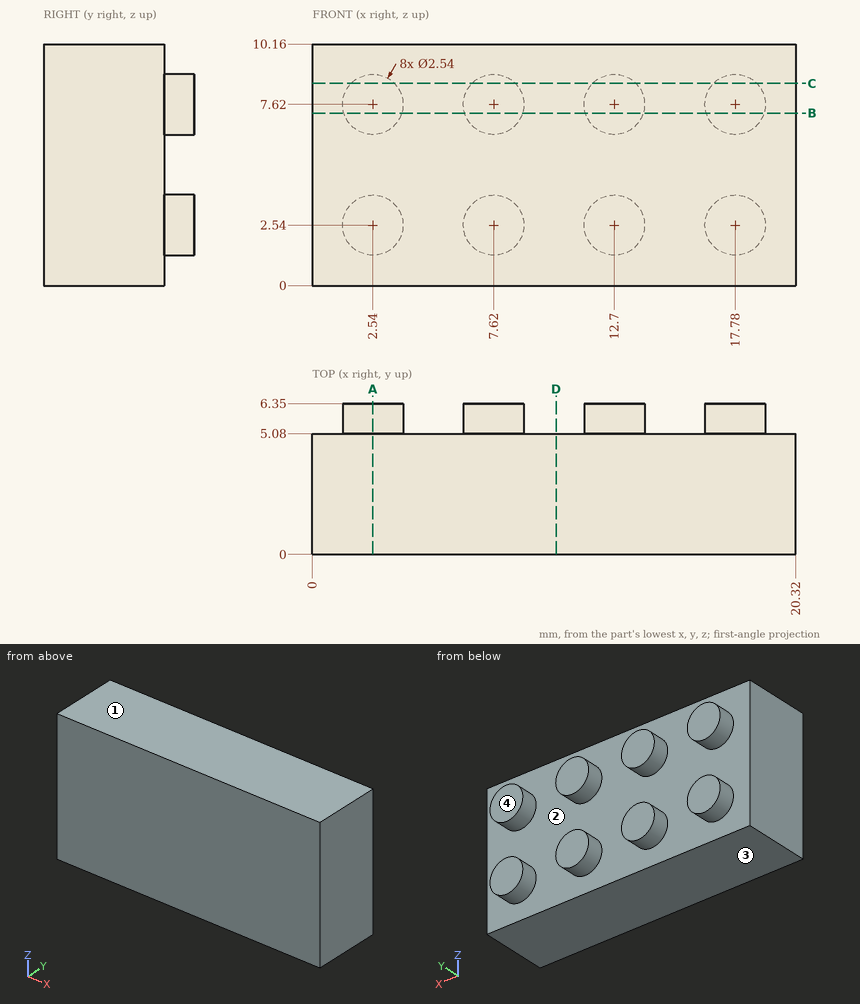
Here's the drawing with two shaded views (mm, measured from the low corner). I have some questions. Coordinates: 2 decimals unless noted, no trailing zeros. Loops run counter-clockwise (first coordinate to the right, second up) from the corner with the lowest first, then second, coordinate; pieces in that order, holes last.
Item 1: Suppose I cut it at C-C (z = 8.5). Please give me the cut outline in (x, y), then the cut area to 3 significant figures.
Answers below:
outline: (0, 0) - (20.32, 0) - (20.32, 5.08) - (18.7, 5.08) - (18.7, 6.35) - (16.86, 6.35) - (16.86, 5.08) - (13.62, 5.08) - (13.62, 6.35) - (11.78, 6.35) - (11.78, 5.08) - (8.54, 5.08) - (8.54, 6.35) - (6.7, 6.35) - (6.7, 5.08) - (3.46, 5.08) - (3.46, 6.35) - (1.62, 6.35) - (1.62, 5.08) - (0, 5.08) - close
area: 113 mm2
Item 2: Please list where these lines run through material, in increasing order: L1, parallel to X at y = 5.5, z = 3.5; L2, parallel to Y at x = 9.25, z = 6; L3, parallel to Z at x = 17.25, y = 5.75.
Answers below:
L1: x = 1.71 to 3.37, 6.79 to 8.45, 11.87 to 13.53, 16.95 to 18.61
L2: y = 0 to 5.08
L3: z = 1.39 to 3.69, 6.47 to 8.77
Item 3: If we mould it in two halves opening along Z, with no side actions, what happens to the marked faces 1, 2, 3 and 4? For each: released by +Z, released by -Z, zero draft, split by the parting line, or undercut.
Answers below:
face 1: released by +Z
face 2: undercut
face 3: released by -Z
face 4: zero draft
Item 4: Suppose I cut it at D-D (x = 10.25). Please give me the cut outline in (y, z).
Answers below:
outline: (0, 0) - (5.08, 0) - (5.08, 10.16) - (0, 10.16) - close
Item 5: Suppose I cut it at A-A (x = 2.54). Please give me the cut outline in (y, z), then the cut area to 3 significant figures.
Answers below:
outline: (0, 0) - (5.08, 0) - (5.08, 1.27) - (6.35, 1.27) - (6.35, 3.81) - (5.08, 3.81) - (5.08, 6.35) - (6.35, 6.35) - (6.35, 8.89) - (5.08, 8.89) - (5.08, 10.16) - (0, 10.16) - close
area: 58.1 mm2
Item 6: I'm going to push a flat-ended pin straight in: pin 1 (1.5 mm diameter, centred on x = 5.5, y = 1.5, fed in from -Z). Where does the tip first touch, or does it pass through?
Answers below:
pin 1: stops at z = 0
Item 7: Suppose I cut it at B-B (z = 7.25). Please give me the cut outline in (x, y), then the cut area to 3 significant figures.
Answers below:
outline: (0, 0) - (20.32, 0) - (20.32, 5.08) - (18.99, 5.08) - (18.99, 6.35) - (16.57, 6.35) - (16.57, 5.08) - (13.91, 5.08) - (13.91, 6.35) - (11.49, 6.35) - (11.49, 5.08) - (8.83, 5.08) - (8.83, 6.35) - (6.41, 6.35) - (6.41, 5.08) - (3.75, 5.08) - (3.75, 6.35) - (1.33, 6.35) - (1.33, 5.08) - (0, 5.08) - close
area: 116 mm2
